Verification items for this drawing (mm, ordinates from the low corner). Give positions to 0.01 mm unless a question says otherwise; leave off trailing zeros. Loops run counter-clockwise (first coordinate to the right, second up) from the corner with the lowest first, then second, coordinate; pieces in that order, holes last. Notation, with made-up numbers: (57.5, 52.25) -> (73.5, 52.25) arc R18 cw to (73.5, 56.25) -> close; hole circle Ø8 at (73, -4). An arc over 180 degrees is marked (long way). Write each question's results on one line, items separated by ' | '. Start each with the question number.
Item 1: Cross-section at B-B on x = 73. Enter the section's corners in (y, z), then the cut area to 3 significant figures.
Item 2: Scan lines: line 1 along X through (y, z) = (13.75, 2.95); line 2 along X through (y, z) = (10, 2.15); line 3 along Y through (x, z) = (162.5, 2.35). Record each from-to range of solid material in increasing order.
Item 3: Cross-section at A-A on z = 0.8. Enter the section's corners in (x, y).
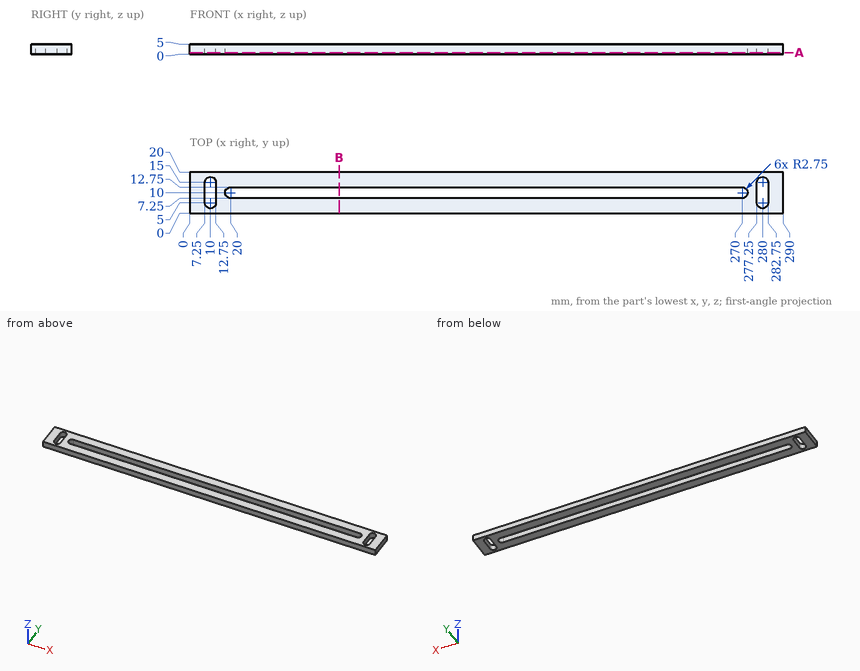
Answer sheet:
1) outline: (0, 0) -> (7.25, 0) -> (7.25, 5) -> (0, 5) -> close; (12.75, 0) -> (20, 0) -> (20, 5) -> (12.75, 5) -> close | area: 72.5 mm²
2) line 1: x = 0 to 7.25, 12.75 to 277.25, 282.75 to 290 | line 2: x = 0 to 7.25, 12.75 to 17.25, 272.75 to 277.25, 282.75 to 290 | line 3: y = 0 to 7.25, 12.75 to 20
3) outline: (0, 0) -> (290, 0) -> (290, 20) -> (0, 20) -> close; hole (7.25, 5) arc R2.75 ccw to (12.75, 5) -> (12.75, 15) arc R2.75 ccw to (7.25, 15) -> close; hole (20, 7.25) -> (270, 7.25) arc R2.75 ccw to (270, 12.75) -> (20, 12.75) arc R2.75 ccw to start; hole (277.25, 5) arc R2.75 ccw to (282.75, 5) -> (282.75, 15) arc R2.75 ccw to (277.25, 15) -> close
